Read the model definition and answer for the solid it produces. Units are mm, in the model's axes. A direction names the side the tool comes from. Coordinates: 2 decimals unless noted, no trailing zeros. Write each loop counter-clockwise with the first axis right and the second up, starting at its lowest first coordinate (ties: lowest second). Pieces come first, ordered by that corner, then holes. Notation, with made-up numbers: (43, 19.5) - (102, 19.5) arc R20 ccw to (102, 24.5) - close; hole circle Ø1 at (-25.5, 11.5). An arc over 180 degrees is marked (long way). Use a Markdown table: item, result.
from build123d import *

# Parameters (mm, degrees)
SKETCH2_R               = 11.049
SKETCH2_R_2             = 10.414
BOSS_EXTRUDE1_DEPTH     = 5.08
SKETCH5_W               = 17.78
SKETCH5_H               = 25.4
SKETCH5_H_2             = 6.490496921
CUT_EXTRUDE2_DEPTH      = 154.417080826
SKETCH3_R               = 8.8265
CUT_EXTRUDE3_DEPTH      = 6.35
SKETCH6_R               = 1.905
CUT_EXTRUDE4_DEPTH      = 164.418972888
CUT_EXTRUDE4_DEPTH_BACK = 164.418972888


with BuildPart() as part:
    # Sketch1 → Revolve1 (revolve)
    with BuildSketch(Plane.XY, mode=Mode.PRIVATE) as revolve1_sk:
        with BuildLine():
            Line((0, 11.320953756), (-10.414, 11.320953756))
            Line((-10.414, 11.320953756), (-5.358147253, -147.429046244))
            ThreePointArc((-5.358147253, -147.429046244), (-3.729882948, -151.108963516), (0, -152.619264469))
            Line((0, -152.619264469), (0, 11.320953756))
        make_face()
    revolve(revolve1_sk.sketch.rotate(Axis((0, 11.320953756, 0), (0, -1, 0)), 180), axis=Axis((0, 11.320953756, 0), (0, -1, 0)))

    # Sketch2 → Boss-Extrude1 (add)
    with BuildSketch(Plane(origin=(0, 11.320953756, 0), x_dir=(1, 0, 0), z_dir=(0, 1, 0))):
        with Locations(Location((0, 0, 0), (0, 0, 270))):
            Circle(SKETCH2_R)
        Circle(SKETCH2_R_2, mode=Mode.SUBTRACT)
        Circle(SKETCH2_R_2)
    extrude(amount=BOSS_EXTRUDE1_DEPTH)

    # Sketch5 → Cut-Extrude2 (cut, through all)
    with BuildSketch(Plane(origin=(0, 0, 0), x_dir=(0, 0, -1), z_dir=(1, 0, 0))):
        with Locations((-5.234813406, -17.889046244)):
            Rectangle(SKETCH5_W, SKETCH5_H)
        with Locations((-5.234813406, -81.389046244)):
            Rectangle(SKETCH5_W, SKETCH5_H)
        with Locations((-5.234813406, -135.434294705)):
            Rectangle(SKETCH5_W, SKETCH5_H_2)
    extrude(amount=-CUT_EXTRUDE2_DEPTH, mode=Mode.SUBTRACT)

    # Sketch3 → Cut-Extrude3 (cut)
    with BuildSketch(Plane(origin=(0, 16.400953756, 0), x_dir=(1, 0, 0), z_dir=(0, 1, 0))):
        with Locations(Location((0, 0, 0), (0, 0, 270))):
            Circle(SKETCH3_R)
    extrude(amount=-CUT_EXTRUDE3_DEPTH, mode=Mode.SUBTRACT)

    # Sketch6 → Cut-Extrude4 (cut, two sides)
    with BuildSketch(Plane(origin=(0, 10.050953756, 0), x_dir=(1, 0, 0), z_dir=(0, 1, 0))) as cut_extrude4_sk:
        with Locations(Location((0, 0, 0), (0, 0, 270))):
            Circle(SKETCH6_R)
    extrude(amount=CUT_EXTRUDE4_DEPTH, mode=Mode.SUBTRACT)
    extrude(cut_extrude4_sk.sketch, amount=-CUT_EXTRUDE4_DEPTH_BACK, mode=Mode.SUBTRACT)


solid = part.part
(1) Straight lines are drawn through the part: L1, parallel to X at y = 12.25, z = 0; L2, parallel to Y at x = -3.5, z = 0.75; L3, parallel to X at y = -141.5, z = 0.75. For each, find the intervals that lie inside material, in ascending order.
Report:
| item | result |
|---|---|
| L1 | x = -11.05 to -8.83, 8.83 to 11.05 |
| L2 | y = -151.25 to -138.68, -132.19 to -94.09, -68.69 to -30.59, -5.19 to 10.05 |
| L3 | x = -5.5 to -1.75, 1.75 to 5.5 |
(2) Each of these flat-tipped pins is pushed along its axis until it touches: P1, Ø6.5, axis at y = -85, z = 4.5, coming from the -X side; P2, Ø12, axis at x = 2, z = -8, coming from the -Y side; P3, Ø8, axis at x = 2, y = -4.5, coming from the +Z side. Where does it stop, or does it pass through?
Report:
| item | result |
|---|---|
| P1 | stops at x = 0 |
| P2 | stops at y = -152.13 |
| P3 | stops at z = 10.02 |
(3) For faces 1 (the flat face through (-3, -94.089, 2)), 2 (the flat face through (-9, 16.401, -1)), 3 (the cylindrical face through (8.75, 13.27, -1.15)), 4 (the conical face through (7.25, -69.17, -3.01)), determine the directions among +Z, -Z, +X, -X, +Y, -Y from which every point of the face is accessible in a straight line to the end or side of a thin tool.
Report:
| item | result |
|---|---|
| face 1 | +Z, -X |
| face 2 | +Z, -Z, +X, -X, +Y |
| face 3 | +Y |
| face 4 | -Y |
(4) The mould has two halves that part along Z. Classify faces 5 (the flat face through (2.1, 10.051, -0.1)), 6 (the flat face through (-2, -135, -3.655)), 7 (the cylindrical face through (1.89, -69.97, -0.25)), 8 (the flat face through (0, -135, 4)): pulls with the +Z half, pulls with the -Z half, needs draft (parallel to the pull), parting line crosses it, or undercut.
Report:
| item | result |
|---|---|
| face 5 | undercut |
| face 6 | pulls with the +Z half |
| face 7 | undercut |
| face 8 | needs draft |
(5) A cutting plane is placed at C-C, the plane y = -74.5. Write down the section's boundary in (x, z) (3 decimals), and give its area (3 significant figures).
Report:
| item | result |
|---|---|
| outline | (-6.755, -3.655) arc R7.681 ccw (long way) to (0, 7.681) - (0, 1.905) arc R1.905 cw to (0, -1.905) - (0, -3.655) - close |
| area | 106 mm² |
(6) A cutting plane is placed at B-B, the plane y = -125. Write down the section's boundary in (x, z) (3 decimals).
Report:
| item | result |
|---|---|
| outline | circle Ø12.145 at (0, 0); hole circle Ø3.81 at (0, 0) |
(7) A cutting plane is placed at A-A, the plane z = 0. Write down the section's boundary in (x, y) (1 decimal).
Report:
| item | result |
|---|---|
| outline | (-11, 11.3) - (-10.4, 11.3) - (-9.9, -5.2) - (-1.9, -5.2) - (-1.9, 10.1) - (-8.8, 10.1) - (-8.8, 16.4) - (-11, 16.4) - close; (-9.1, -30.6) - (-7.9, -68.7) - (-1.9, -68.7) - (-1.9, -30.6) - close; (-7.1, -94.1) - (-5.8, -132.2) - (-1.9, -132.2) - (-1.9, -94.1) - close; (-5.6, -138.7) - (-5.4, -147.4) arc R5.4 ccw to (-1.9, -152.3) - (-1.9, -138.7) - close; (1.9, -152.3) arc R5.4 ccw to (5.4, -147.4) - (10.4, 11.3) - (11, 11.3) - (11, 16.4) - (8.8, 16.4) - (8.8, 10.1) - (1.9, 10.1) - close |
